```python
from build123d import *

# Parameters (mm, degrees)
SKETCH_1_R             = 1.75
SKETCH_1_R_2           = 1
SM_BASE_FLANGE_1_DEPTH = 1.2


# Sheet-metal steps are written as plain solids
with BuildPart() as part:
    # Sketch 1 → Базовая кромка1 (new body)
    with BuildSketch(Plane.XY):
        Polygon((0, 0), (12, 0), (12, 5), (8, 5), (8, 20), (0, 20), align=None)
        with Locations((4, 16)):
            Circle(SKETCH_1_R, mode=Mode.SUBTRACT)
        with Locations((4, 9.5)):
            Circle(SKETCH_1_R_2, mode=Mode.SUBTRACT)
        with Locations((4, 3.9)):
            Circle(SKETCH_1_R_2, mode=Mode.SUBTRACT)
    extrude(amount=-SM_BASE_FLANGE_1_DEPTH)


solid = part.part
```
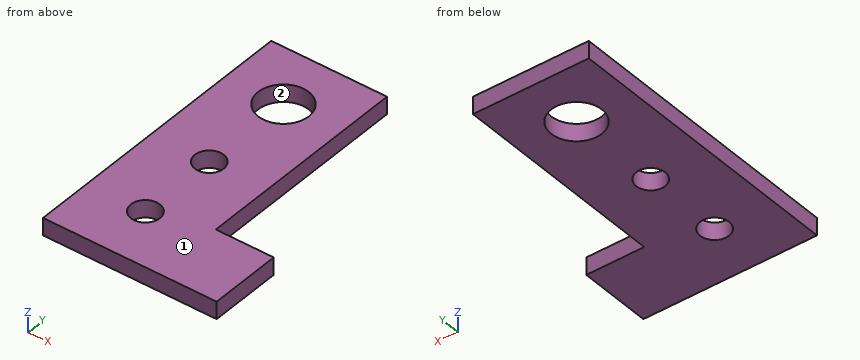
Build history of the part. All positions in model axes, mm. Face numbers are marked on the shaded views. Give positions to 0.01 mm unless a question says otherwise; leave off trailing zeros. Order: outer loops, then holes, each group sorted by start corner. A loop starts at its lowest first (then second) coordinate and runs counter-clockwise, first axis right, second up. Notation, with made-up numbers: M 41.5,89.25 L 88.5,89.25 A21 cw 88.5,96.25 Z; hole C 34.25,34 d1. An arc over 180 degrees is marked long. Return JSON: item names as keys, results as strings.
Q1. Band-saw the part on B-B (x = 4). Give the cut face in (y, z), then the cut area to 3 significant figures.
Answer list:
{"outline": "M 0,-1.2 L 2.9,-1.2 L 2.9,0 L 0,0 Z; M 4.9,-1.2 L 8.5,-1.2 L 8.5,0 L 4.9,0 Z; M 10.5,-1.2 L 14.25,-1.2 L 14.25,0 L 10.5,0 Z; M 17.75,-1.2 L 20,-1.2 L 20,0 L 17.75,0 Z", "area": "15.0 mm^2"}
Q2. Band-saw the part on A-A (y = 4.5). Give the cut face in (x, z).
Answer list:
{"outline": "M 0,-1.2 L 3.2,-1.2 L 3.2,0 L 0,0 Z; M 4.8,-1.2 L 12,-1.2 L 12,0 L 4.8,0 Z"}
Q3. Wall check: probe 1 along Y at (x, z) = (4, -0.3); probe 2 along Y at (x, z) = (3.5, -0.5); probe 3 along X at (y, z) = (12.5, -0.35). Give the ranges that are in metal, low to high. Write a range as from..to.
Answer list:
{"probe 1": "y = 0..2.9, 4.9..8.5, 10.5..14.25, 17.75..20", "probe 2": "y = 0..3.03, 4.77..8.63, 10.37..14.32, 17.68..20", "probe 3": "x = 0..8"}
Q4. Two-plate mould, pull along X, no slides. Class the marked faces 1 and 2: pulls with the +X half, pulls with the -X half, needs draft (parallel to the pull), parting line crosses it, or undercut.
Answer list:
{"face 1": "needs draft", "face 2": "undercut"}
Q5. Band-saw the part on D-D (y = 16). Give the cut face in (x, z).
Answer list:
{"outline": "M 0,-1.2 L 2.25,-1.2 L 2.25,0 L 0,0 Z; M 5.75,-1.2 L 8,-1.2 L 8,0 L 5.75,0 Z"}
Q6. Band-saw the part on C-C (z = -0.95). Give the cut face in (x, y), then the cut area to 3 significant figures.
Answer list:
{"outline": "M 0,0 L 12,0 L 12,5 L 8,5 L 8,20 L 0,20 Z; hole C 4,16 d3.5; hole C 4,3.9 d2; hole C 4,9.5 d2", "area": "164 mm^2"}
